Geometry: final body of the model. Coordinates: model frame, mm. Round coordinates to 2 decimals unless told otherwise and drop trailing zeros. Loops run counter-clockwise (first coordinate to the right, second up) from the corner with the lowest first, then second, coordinate; pieces in that order, holes last. Notation, with made-up numbers: M 8.5,-10.5 L 45.5,-10.5 A16 ccw 45.5,10.5 Z; hole C -7,-6 d6. An arc over 180 degrees is marked long. Answer as a JSON object with one key per item and string values.
Autodesk Inventor part; units mm, degrees
ref_plane "YZ Plane" through (0, 0, 0) normal (1, 0, 0) x (0, 1, 0)
ref_plane "XZ Plane" through (0, 0, 0) normal (0, 1, 0) x (-1, 0, 0)
ref_plane "XY Plane" through (0, 0, 0) normal (0, 0, 1) x (1, 0, 0)
sketch "Эскиз1" plane through (0, 0, 0) normal (0, 0, 1) x (1, 0, 0)
  line L0 (4.75, 0) -> (13, 0)
  line L1 (13, 0) -> (13, 1.5)
  line L2 (13, 1.5) -> (4.75, 1.5)
  line L3 (0, 1.5) -> (0, 0)
  line L4 (4.75, 1.5) -> (4.75, 0)
  dimension "d0" = 26
  dimension "d3" = 1.5
  dimension "d7" = 9.5
revolve "Вращение1" add sketch "Эскиз1" angle 360 about axis through (0, 1.5, 0) along (0, -1, 0)
fillet "Сопряжение3" radius 0.4 4 edges at (-13, 0, 0) (-13, 1.5, 0) (-4.75, 0, 0) (-4.75, 1.5, 0)
equation "\"d3\" = d2"
properties part number "paris_washer"
1) Pull-direction query (Z, two-part tool) for faces 1 (the flat face through (5.4, 0, 0.2)), 2 (the cylindrical face through (-10.316, 0.755, 7.91)), 3 (the cylindrical face through (2.192, 0.745, -4.214)); classes: +Z half, -Z half, draft (parallel to the pull), parting line (faces both ways), or undercut.
Results:
{"face 1": "draft", "face 2": "parting line", "face 3": "undercut"}
2) Section query B-B (z = 0). Return the cut outline in (x, y), and give its area (3 significant figures).
Results:
{"outline": "M -13,0.4 A0.4 ccw -12.6,0 L -5.15,0 A0.4 ccw -4.75,0.4 L -4.75,1.1 A0.4 ccw -5.15,1.5 L -12.6,1.5 A0.4 ccw -13,1.1 Z; M 4.75,0.4 A0.4 ccw 5.15,0 L 12.6,0 A0.4 ccw 13,0.4 L 13,1.1 A0.4 ccw 12.6,1.5 L 5.15,1.5 A0.4 ccw 4.75,1.1 Z", "area": "24.5 mm2"}
3) Ray query, line 1 (Z direction, x = 0, y = 0.65); line 2 (X direction, y = 0.35, z = -0.25); line 3 (Z direction, x = -2.25, y = 0.8). Return the intervals inside material, ascending.
Results:
{"line 1": "-13 to -4.75, 4.75 to 13", "line 2": "-12.99 to -4.75, 4.75 to 12.99", "line 3": "-12.8 to -4.18, 4.18 to 12.8"}
4) Section query A-A (x = 0). Return the cut outline in (y, z).
Results:
{"outline": "M 0,-12.6 A0.4 ccw 0.4,-13 L 1.1,-13 A0.4 ccw 1.5,-12.6 L 1.5,-5.15 A0.4 ccw 1.1,-4.75 L 0.4,-4.75 A0.4 ccw 0,-5.15 Z; M 0,5.15 A0.4 ccw 0.4,4.75 L 1.1,4.75 A0.4 ccw 1.5,5.15 L 1.5,12.6 A0.4 ccw 1.1,13 L 0.4,13 A0.4 ccw 0,12.6 Z"}
5) Section query C-C (y = 0.8). Return the cut outline in (x, z).
Results:
{"outline": "C 0,0 d26; hole C 0,0 d9.5"}
